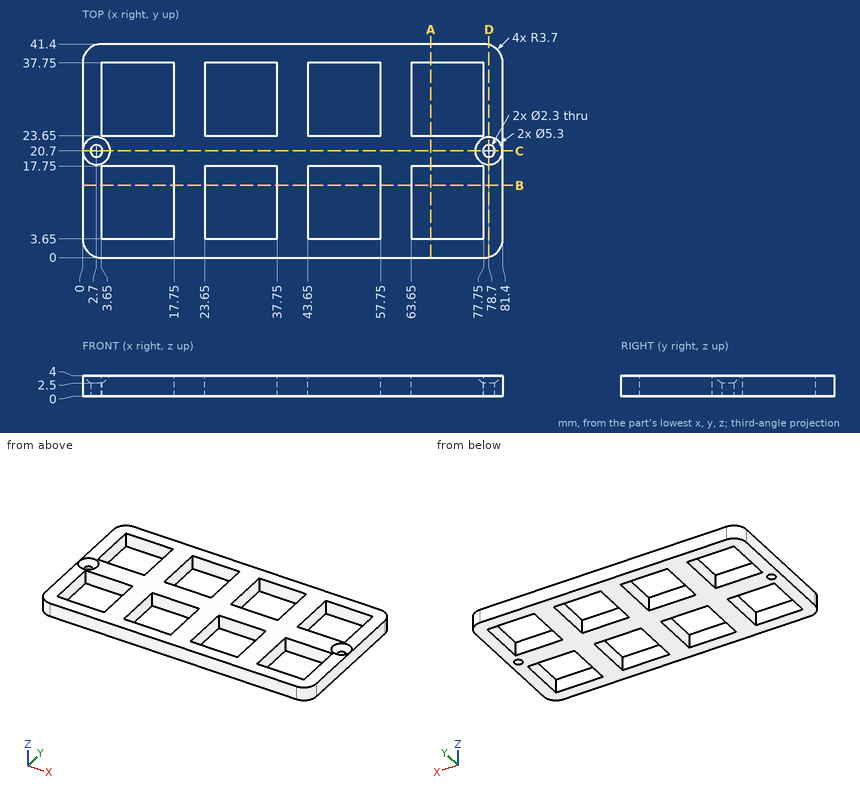
The drawing under review shows one solid part. Ordinate dimensions are in mm from its lowest x, y, z. Round coordinates to 2 decimals unless told otherwise and drop trailing zeros. Write each loop counter-clockwise with the first axis right and the second up, starting at its lowest first coordinate (ties: lowest second). Pieces come first, ordered by that corner, then holes. Notation, with made-up numbers: (2.25, 79) -> (53.25, 79) arc R19 cw to (53.25, 89) -> close; hole circle Ø10 at (58, 41). An arc over 180 degrees is marked (long way). One line per question, with ' | ' between items. Start each with the question number.
(1) For line 1 along Y through (x, z) = (9, 1.5); line 2 along X through (y, z) = (31, 1.3); line 3 along Y through (x, z) = (78.7, 0.8), list the stretches that pass through material, from the lowest coordinate up. Write a range as from..to.
(2) Add section A-A, the plane x = 67.5. Write out the cut boundary in (y, z), plus the area to 3 significant figures.
(3) Insertion check: P1, Ø1.4, axis at x = 2.7, y = 20.7, coming from the -Z side. The pin has a flat end and moves straight along its axis. Give the tip position at first contact, or say it passes through.
(4) Add section C-C, the plane y = 20.7. Write out the cut boundary in (x, z).
(5) Add section B-B, the plane y = 14. Write out the cut boundary in (x, z), plus the area to 3 significant figures.
(6) Add section D-D, the plane x = 78.7. Write out the cut boundary in (y, z).
Answer list:
1) line 1: 0..3.65, 17.75..23.65, 37.75..41.4 | line 2: 0..3.65, 17.75..23.65, 37.75..43.65, 57.75..63.65, 77.75..81.4 | line 3: 0.14..19.55, 21.85..41.26
2) outline: (0, 0) -> (3.65, 0) -> (3.65, 4) -> (0, 4) -> close; (17.75, 0) -> (23.65, 0) -> (23.65, 4) -> (17.75, 4) -> close; (37.75, 0) -> (41.4, 0) -> (41.4, 4) -> (37.75, 4) -> close | area: 52.8 mm²
3) P1: through
4) outline: (0, 0) -> (1.55, 0) -> (1.55, 2.5) -> (0.05, 4) -> (0, 4) -> close; (3.85, 0) -> (77.55, 0) -> (77.55, 2.5) -> (76.05, 4) -> (5.35, 4) -> (3.85, 2.5) -> close; (79.85, 0) -> (81.4, 0) -> (81.4, 4) -> (81.35, 4) -> (79.85, 2.5) -> close
5) outline: (0, 0) -> (3.65, 0) -> (3.65, 4) -> (0, 4) -> close; (17.75, 0) -> (23.65, 0) -> (23.65, 4) -> (17.75, 4) -> close; (37.75, 0) -> (43.65, 0) -> (43.65, 4) -> (37.75, 4) -> close; (57.75, 0) -> (63.65, 0) -> (63.65, 4) -> (57.75, 4) -> close; (77.75, 0) -> (81.4, 0) -> (81.4, 4) -> (77.75, 4) -> close | area: 100 mm²
6) outline: (0.14, 0) -> (19.55, 0) -> (19.55, 2.5) -> (18.05, 4) -> (0.14, 4) -> close; (21.85, 0) -> (41.26, 0) -> (41.26, 4) -> (23.35, 4) -> (21.85, 2.5) -> close
